Source: CAD feature listing. Evaluate the final solid. Frame: model axes, mm. A direction names the side the tool comes from. Give positions to 0.01 mm unless a question says otherwise; leave off trailing zeros. Write each loop counter-clockwise with the first axis right and the second up, starting at its lowest first coordinate (ties: lowest second). Pieces come first, ordered by that corner, then holes. Notation, with made-up numbers: (16, 62) -> (69, 62) arc R29 ccw to (69, 96) -> close; hole circle Ø10 at (0, 58). An arc over 180 degrees is marked (long way). Use one line per item in the form item = value. Start each with the question number.
(1) Cut plane B-B, the plane y = -50. Output: boundary loops of the cut face in (x, z).
(2) Cut plane C-C, the plane z = -41. Output: boundary loops of the cut face in (x, y) (3 decimals), and give its area (3 significant figures).
(3) Cut plane D-D, the plane x = -20.5. Output: boundary loops of the cut face in (y, z), and give its area (3 significant figures).
(4) Draft query along Z for faces 1 (the face through (0, -20, 38.1)), 2 (the face through (-5.506, -79.331, -24.796)), 3 (the face through (0, -25, 50.8)), 4 (the face through (-25.4, -66, 0)). Return one class per face: pulls with the +Z half, pulls with the -Z half, needs draft (parallel to the pull), parting line crosses it, or undercut.
(5) Material intervals for line 1 along Z through (x, y) = (16, 0.5); line 2 along Y through (x, z) = (0, -46) (3 decimals); line 3 along Y through (x, z) = (19, -18.5), sorted ascending. Write a range as from..to.
(6) Set-up query: faces 5 (the face through (0, -25, -50.8)), 6 (the face through (0, -20, -38.1)), 7 (the face through (0, -76.2, -36)). Return all of +Z, -Z, +X, -X, +Y, -Y with unobstructed straight access to the full face (end or side cutting, diameter ignored); none if empty.
(7) First-contact query: P1, Ø1, axis at x = 2, z = -33.5, coming from the -Y side; P2, Ø3, axis at x = -7, z = -22, coming from the +Y side; P3, Ø10, axis at x = 4.5, z = 38.5, coming from the +Y side. Flat tips, straight axial feed; report the tip coordinate or a pass-through.
(8) Cut plane A-A, the plane x = 0. Output: boundary loops of the cut face in (y, z) (3 decimals), and give its area (3 significant figures).
from build123d import *

# Parameters (mm, degrees)
SKETCH1_R               = 9.525
BOSS_EXTRUDE1_DEPTH     = 50.8
SKETCH2_W               = 76.2
SKETCH2_H               = 88.9
CUT_EXTRUDE1_DEPTH      = 26.4
CUT_EXTRUDE1_DEPTH_BACK = 26.4
SKETCH3_R               = 25.4
BOSS_EXTRUDE2_DEPTH     = 6.35


with BuildPart() as part:
    # Sketch1 → Boss-Extrude1 (new body, symmetric)
    with BuildSketch(Plane.XY):
        with BuildLine():
            Line((-25.4, 0), (-25.4, -76.2))
            Line((-25.4, -76.2), (25.4, -76.2))
            Line((25.4, -76.2), (25.4, 0))
            ThreePointArc((25.4, 0), (0, 25.4), (-25.4, 0))
        make_face()
        Circle(SKETCH1_R, mode=Mode.SUBTRACT)
    extrude(amount=BOSS_EXTRUDE1_DEPTH, both=True)

    # Sketch2 → Cut-Extrude1 (cut, two sides)
    with BuildSketch(Plane(origin=(0, 0, 0), x_dir=(0, 0, -1), z_dir=(1, 0, 0))) as cut_extrude1_sk:
        with Locations((0, -19.05)):
            Rectangle(SKETCH2_W, SKETCH2_H)
    extrude(amount=CUT_EXTRUDE1_DEPTH, mode=Mode.SUBTRACT)
    extrude(cut_extrude1_sk.sketch, amount=-CUT_EXTRUDE1_DEPTH_BACK, mode=Mode.SUBTRACT)

    # Sketch3 → Boss-Extrude2 (add)
    with BuildSketch(Plane.XZ.offset(76.2)):
        Circle(SKETCH3_R)
    extrude(amount=BOSS_EXTRUDE2_DEPTH)


solid = part.part
Geometry says:
q1.outline = (-25.4, -50.8) -> (25.4, -50.8) -> (25.4, -38.1) -> (-25.4, -38.1) -> close; (-25.4, 38.1) -> (25.4, 38.1) -> (25.4, 50.8) -> (-25.4, 50.8) -> close
q2.outline = (-25.4, -76.2) -> (25.4, -76.2) -> (25.4, 0) arc R25.4 ccw to (-25.4, 0) -> close; hole circle Ø19.05 at (0, 0)
q2.area = 4,600 mm^2
q3.outline = (-82.55, -15) -> (-76.2, -15) -> (-76.2, -50.8) -> (15, -50.8) -> (15, -38.1) -> (-63.5, -38.1) -> (-63.5, 38.1) -> (15, 38.1) -> (15, 50.8) -> (-76.2, 50.8) -> (-76.2, 15) -> (-82.55, 15) -> close
q3.area = 3,470 mm^2
q4.face_1 = undercut
q4.face_2 = parting line crosses it
q4.face_3 = pulls with the +Z half
q4.face_4 = needs draft
q5.line_1 = -50.8..-38.1, 38.1..50.8
q5.line_2 = -76.2..-9.525, 9.525..25.4
q5.line_3 = -76.2..-63.5
q6.face_5 = -Z, +X, -X, +Y, -Y
q6.face_6 = +X, -X, +Y
q6.face_7 = -Z, -Y
q7.P1 = -76.2
q7.P2 = -63.5
q7.P3 = 25.4
q8.outline = (-82.55, -25.4) -> (-76.2, -25.4) -> (-76.2, -50.8) -> (-9.525, -50.8) -> (-9.525, -38.1) -> (-63.5, -38.1) -> (-63.5, 38.1) -> (-9.525, 38.1) -> (-9.525, 50.8) -> (-76.2, 50.8) -> (-76.2, 25.4) -> (-82.55, 25.4) -> close; (9.525, -50.8) -> (25.4, -50.8) -> (25.4, -38.1) -> (9.525, -38.1) -> close; (9.525, 38.1) -> (25.4, 38.1) -> (25.4, 50.8) -> (9.525, 50.8) -> close
q8.area = 3,390 mm^2
